```python
from build123d import *

# Parameters (mm, degrees)
CYLINDER032_R     = 15
CYLINDER032_DEPTH = 25
CYLINDER030_R     = 100
CYLINDER030_DEPTH = 25
CYLINDER031_R     = 15
CYLINDER031_DEPTH = 25
BOX008_W          = 160
BOX008_H          = 30
BOX008_DEPTH      = 25
FILLET034_R       = 4


with BuildPart() as cylinder032:
    # Cylinder032 → Cylinder032 (new body)
    with BuildSketch(Plane(origin=(55, -107, 0), x_dir=(1, 0, 0), z_dir=(0, 0, 1))):
        Circle(CYLINDER032_R)
    extrude(amount=CYLINDER032_DEPTH)


with BuildPart() as cylinder030:
    # Cylinder030 → Cylinder030 (new body)
    with BuildSketch(Plane(origin=(0, 1.5, 0), x_dir=(1, 0, 0), z_dir=(0, 0, 1))):
        Circle(CYLINDER030_R)
    extrude(amount=CYLINDER030_DEPTH)


with BuildPart() as fusion013:
    # Cylinder031 → Cylinder031 (new body)
    with BuildSketch(Plane(origin=(-55, -107, 0), x_dir=(1, 0, 0), z_dir=(0, 0, 1))):
        Circle(CYLINDER031_R)
    extrude(amount=CYLINDER031_DEPTH)

    # Fusion013: union Cylinder032, Cylinder030
    add(cylinder032.part)
    add(cylinder030.part)


with BuildPart() as holder:
    # Box008 → Box008 (new body)
    with BuildSketch(Plane(origin=(-80, -100, 0), x_dir=(1, 0, 0), z_dir=(0, 0, 1))):
        with Locations((80, 15)):
            Rectangle(BOX008_W, BOX008_H)
    extrude(amount=BOX008_DEPTH)

    # Cut020: cut Fusion013
    add(fusion013.part, mode=Mode.SUBTRACT)

    # Fillet034
    fillet034_edges = [holder.edges().sort_by_distance(p)[0] for p in [
        (-80, -100, 12.5),
        (-80, -70, 12.5),
        (-68.266499, -100, 12.5),
        (80, -70, 12.5),
        (80, -100, 12.5),
        (68.266499, -100, 12.5),
    ]]
    fillet(fillet034_edges, radius=FILLET034_R)


solid = holder.part
```
Could you check a few things on this model? Use its own coordinates, in mm. A direction names the side the tool comes from. Give positions to 0.01 mm unless a question says otherwise; leave off trailing zeros. Loops run counter-clockwise (first coordinate to the right, second up) from the corner with the lowest first, then second, coordinate; pieces in that order, holes last. Notation, with made-up numbers: (-14.5, -20) - (28.5, -20) arc R10 ccw to (28.5, -5) - close; hole circle Ø9 at (-21.75, -39.75). An arc over 180 degrees is marked (long way). Answer in a Markdown table with one row per item. Add a question column.
Q1. Please list where these lines run through material, in increasing order: L1, parallel to X at y = -76.5, z = 16.25; L2, parallel to X at y = -74, z = 1.25; L3, parallel to Y at x = 15, z = 16.75. Write a range as from..to.
Q2. If we section it at C-C (y = -82): List the corners of the cut face in (x, z) for me (3 decimals), plus the area to 3 significant figures.
Q3. If we section it at A-A (y = -90): List the corners of the cut face in (x, z) for me, plus the area to 3 significant figures.
Q4. We'd pull the mould along X, two halves only. Please class faces 1 (the face through (-1.084, -98.494, 12.325)), 2 (the face through (-73, -70, 12)), 3 (the face through (54.23, -92.02, 12.32)), 4 (the face through (-78.859, -71.203, 12.675)): +X half, -X half, draft (parallel to the pull), parting line (faces both ways), or undercut.
Q5. If we section it at B-B (z = 23): List the corners of the cut face in (x, y) for me, plus the area to 3 significant figures.
Q6. For pin 1 (3 mm diameter, centred on x = 20.5, y = -95.5, fed in from +Z); pin 2 (5 mm diameter, centred on x = 45.5, z = 10.5, fed in from +Y); pin 3 (5 mm diameter, centred on x = -25.5, z = 16, fed in from +Y); pin 4 (2 mm diameter, centred on x = 38, z = 15.5, fed in from +Y), each with a flat end and sliding along its axis, tell me the tip position at first contact or that it passes through.
Q7. Which directions (+Z, -Z, +X, -X, +Y, -Y) give clear straight access to the entire face, cutting with the end or side of a thin tool? Please do faces 5 (the face through (-80, -85, 12)), 6 (the face through (-68.68, -99.566, 12.325)).
Q8. If we section it at D-D (x = 51.5): List the corners of the cut face in (y, z) for me, plus the area to 3 significant figures.
The answers:
| question | item | result |
|---|---|---|
| 1 | L1 | x = -80..-62.58, 62.58..80 |
| 1 | L2 | x = -80..-65.57, 65.57..80 |
| 1 | L3 | y = -100..-97.37 |
| 2 | outline | (-80, 0) - (-55.025, 0) - (-55.025, 25) - (-80, 25) - close; (55.025, 0) - (80, 0) - (80, 25) - (55.025, 25) - close |
| 2 | area | 1,250 mm^2 |
| 3 | outline | (-80, 0) - (-40.35, 0) - (-40.35, 25) - (-80, 25) - close; (40.35, 0) - (80, 0) - (80, 25) - (40.35, 25) - close |
| 3 | area | 1,980 mm^2 |
| 4 | face 1 | undercut |
| 4 | face 2 | draft |
| 4 | face 3 | undercut |
| 4 | face 4 | -X half |
| 5 | outline | (-80, -96) arc R4 ccw to (-76, -100) - (-70.49, -100) arc R4 ccw to (-67.23, -98.32) arc R15 cw to (-41.73, -100) - (41.73, -100) arc R15 cw to (67.23, -98.32) arc R4 ccw to (70.49, -100) - (76, -100) arc R4 ccw to (80, -96) - (80, -74) arc R4 ccw to (76, -70) - (69.91, -70) arc R100 cw to (-69.91, -70) - (-76, -70) arc R4 ccw to (-80, -74) - close |
| 5 | area | 1,740 mm^2 |
| 6 | pin 1 | stops at z = 25 |
| 6 | pin 2 | stops at y = -86.23 |
| 6 | pin 3 | stops at y = -94.5 |
| 6 | pin 4 | stops at y = -90.58 |
| 7 | face 5 | +Z, -Z, -X, +Y, -Y |
| 7 | face 6 | +Z, -Z, -Y |
| 8 | outline | (-92.41, 0) - (-84.22, 0) - (-84.22, 25) - (-92.41, 25) - close |
| 8 | area | 205 mm^2 |
